Build history of the part. All positions in model axes, mm. A direction names the side the tool comes from. Give positions to 0.01 mm unless a question says otherwise; leave off trailing zeros. Order: outer loops, then holes, each group sorted by start corner. A loop starts at its lowest first (then second) coordinate and runs counter-clockwise, first axis right, second up. Notation, with made-up numbers: (63, 71.5) - (87, 71.5) arc R19 cw to (87, 83.5) - close; hole circle Ø6 at (39, 72). An arc over 180 degrees is marked (long way). Write each question's results on one line, items separated by ' | '. Start each with the question number.
1) Cut at C-C on x = 25. List the corners of the cut face in (y, z).
2) Drill centre lines: line 1 along Y through (x, z) = (0, 2.5); line 2 along Y through (x, z) = (50, 8.75); line 3 along X through (y, z) = (39, 9.75). Where is each one in solid material? Low to high. Write a range as from..to.
3) Tool access for faces 1 (the face through (62.4, 1, 5)), 2 (the face through (-55.495, -37.742, 3.155)): list every direction of +Z, -Z, +X, -X, +Y, -Y with a clear straight run to the whole face (end or side of a thin tool).
4) Two-plate mould, pull along X, no slides. Class faces 3 (the face through (-28, -12.4, 4.9)), 4 (the face through (-60.596, 48.189, 4.958)), 5 (the face through (60.689, 48.096, 4.958)), 6 (the face through (-27.21, -35.47, 4.93)): +X half, -X half, draft (parallel to the pull), parting line (faces both ways), or undercut.
5) Drop flat-ended pins along their axis: pin 1 Ø9.5 at (x, y) = (-25, -12.5) entering from +Z; pin 2 Ø8.5 at (x, y) = (-50, 37.5) entering from -Z. Give the stop position or say it passes through.
6) Cut at A-A on x = 50. State how many separate pieces and enclosed holes the cut face has, plus the area to 3 significant figures.
from build123d import *

# Parameters (mm, degrees)
SKETCH_R         = 3
PAD_DEPTH        = 10
HOLE_D           = 6.6
HOLE_DEPTH       = 25
HOLE_CBORE_D     = 11
HOLE_CBORE_DEPTH = 6.4
FILLET_R         = 2
FILLET001_R      = 2


with BuildPart() as part:
    # Sketch → Pad (new body)
    with BuildSketch(Plane.XY):
        with BuildLine():
            Line((-56.4, 49.9), (56.4, 49.9))
            ThreePointArc((62.4, 43.9), (60.642641, 48.142641), (56.4, 49.9))
            Line((62.4, 43.9), (62.4, -43.9))
            ThreePointArc((56.4, -49.9), (60.642641, -48.142641), (62.4, -43.9))
            Line((56.4, -49.9), (-56.4, -49.9))
            ThreePointArc((-62.4, -43.9), (-60.642641, -48.142641), (-56.4, -49.9))
            Line((-62.4, -43.9), (-62.4, 43.9))
            ThreePointArc((-56.4, 49.9), (-60.642641, 48.142641), (-62.4, 43.9))
        make_face()
        with Locations((25, -37.5)):
            Circle(SKETCH_R, mode=Mode.SUBTRACT)
        with Locations((0, -37.5)):
            Circle(SKETCH_R, mode=Mode.SUBTRACT)
        with Locations((-25, -37.5)):
            Circle(SKETCH_R, mode=Mode.SUBTRACT)
        with Locations((50, -12.5)):
            Circle(SKETCH_R, mode=Mode.SUBTRACT)
        with Locations((50, 12.5)):
            Circle(SKETCH_R, mode=Mode.SUBTRACT)
        with Locations((-50, -12.5)):
            Circle(SKETCH_R, mode=Mode.SUBTRACT)
        with Locations((-25, -12.5)):
            Circle(SKETCH_R, mode=Mode.SUBTRACT)
        with Locations((0, -12.5)):
            Circle(SKETCH_R, mode=Mode.SUBTRACT)
        with Locations((25, -12.5)):
            Circle(SKETCH_R, mode=Mode.SUBTRACT)
        with Locations((-50, 12.5)):
            Circle(SKETCH_R, mode=Mode.SUBTRACT)
        with Locations((-25, 12.5)):
            Circle(SKETCH_R, mode=Mode.SUBTRACT)
        with Locations((0, 12.5)):
            Circle(SKETCH_R, mode=Mode.SUBTRACT)
        with Locations((25, 12.5)):
            Circle(SKETCH_R, mode=Mode.SUBTRACT)
        with Locations((-25, 37.5)):
            Circle(SKETCH_R, mode=Mode.SUBTRACT)
        with Locations((0, 37.5)):
            Circle(SKETCH_R, mode=Mode.SUBTRACT)
        with Locations((25, 37.5)):
            Circle(SKETCH_R, mode=Mode.SUBTRACT)
    extrude(amount=PAD_DEPTH)

    # Hole
    with Locations(Plane(origin=(0, 0, 0), x_dir=(1, 0, 0), z_dir=(0, 0, -1))):
        with Locations((50, -37.5), (-50, -37.5), (-50, 37.5), (50, 37.5)):
            CounterBoreHole(HOLE_D / 2, HOLE_CBORE_D / 2, HOLE_CBORE_DEPTH, depth=HOLE_DEPTH)

    # Fillet
    fillet_edges = [part.edges().sort_by_distance(p)[0] for p in [
        (0, 49.9, 0),
    ]]
    fillet(fillet_edges, radius=FILLET_R)

    # Fillet001
    fillet001_edges = [part.edges().sort_by_distance(p)[0] for p in [
        (0, 49.9, 10),
    ]]
    fillet(fillet001_edges, radius=FILLET001_R)


solid = part.part
Results:
1) outline: (-49.9, 2) arc R2 ccw to (-47.9, 0) - (-40.5, 0) - (-40.5, 10) - (-47.9, 10) arc R2 ccw to (-49.9, 8) - close; (-34.5, 0) - (-15.5, 0) - (-15.5, 10) - (-34.5, 10) - close; (-9.5, 0) - (9.5, 0) - (9.5, 10) - (-9.5, 10) - close; (15.5, 0) - (34.5, 0) - (34.5, 10) - (15.5, 10) - close; (40.5, 0) - (47.9, 0) arc R2 ccw to (49.9, 2) - (49.9, 8) arc R2 ccw to (47.9, 10) - (40.5, 10) - close
2) line 1: -49.9..-40.5, -34.5..-15.5, -9.5..9.5, 15.5..34.5, 40.5..49.9 | line 2: -49.75..-40.8, -34.2..-15.5, -9.5..9.5, 15.5..34.2, 40.8..49.75 | line 3: -61.37..-52.94, -47.06..-27.6, -22.4..-2.6, 2.6..22.4, 27.6..47.06, 52.94..61.37
3) face 1: +Z, -Z, +X, +Y, -Y | face 2: -Z
4) face 3: undercut | face 4: -X half | face 5: +X half | face 6: undercut
5) pin 1: z = 10 | pin 2: z = 6.4
6) separate pieces: 5 | enclosed holes: 0 | area: 686 mm^2
